Input: dimensioned drawing with shaded views. Units: mm. Origin: part minimum x, y, z. Coordinates: 2 decimals unless noted, no trailing zeros. Order: outer loops, then holes, each group sorted by start corner. A loop starts at its lowest first (then second) coordinate and runs counter-clockwise, first axis right, second up. Notation, with made-up numbers: (87, -10.75) - (104, -10.75) arc R24 ccw to (104, 26.25) - close; hole circle Ø5 at (-33.5, 8). An arc over 180 degrees is marked (long way). One line per question, with ' | ' between items. Start each with the question number.
(1) Section A-A (z = 19.5). Return the cut outline in (x, y).
(2) Section B-B (x = 19.5). Return the cut outline in (y, z), then the cut area to 3 significant figures.
(3) Draft query along Z for the marked faces 1, 2, 3 and 4. Return one class per face: +Z half, -Z half, draft (parallel to the pull), parting line (faces both ways), or undercut.
(4) Line query: line 1 along X through (y, z) = (21.5, 19.5); line 2 along X through (y, z) = (12, 6.5); line 3 along Z through (x, y) = (12.5, 22). Output: solid intervals per line, ascending.
(5) Section D-D (y = 3). Return the cut outline in (x, z).
(6) Section C-C (y = 11). Return the cut outline in (x, z).
(7) Contact query for flat-ended pins moving along their axis: P1, Ø1.5, axis at x = 32.5, z = 16, coming from the -Y side; P2, Ø6, axis at y = 6, z = 14.5, coming from the -X side; P3, Ø4, axis at x = 19, z = 21, coming from the +Y side. Output: stop coordinate, or through.
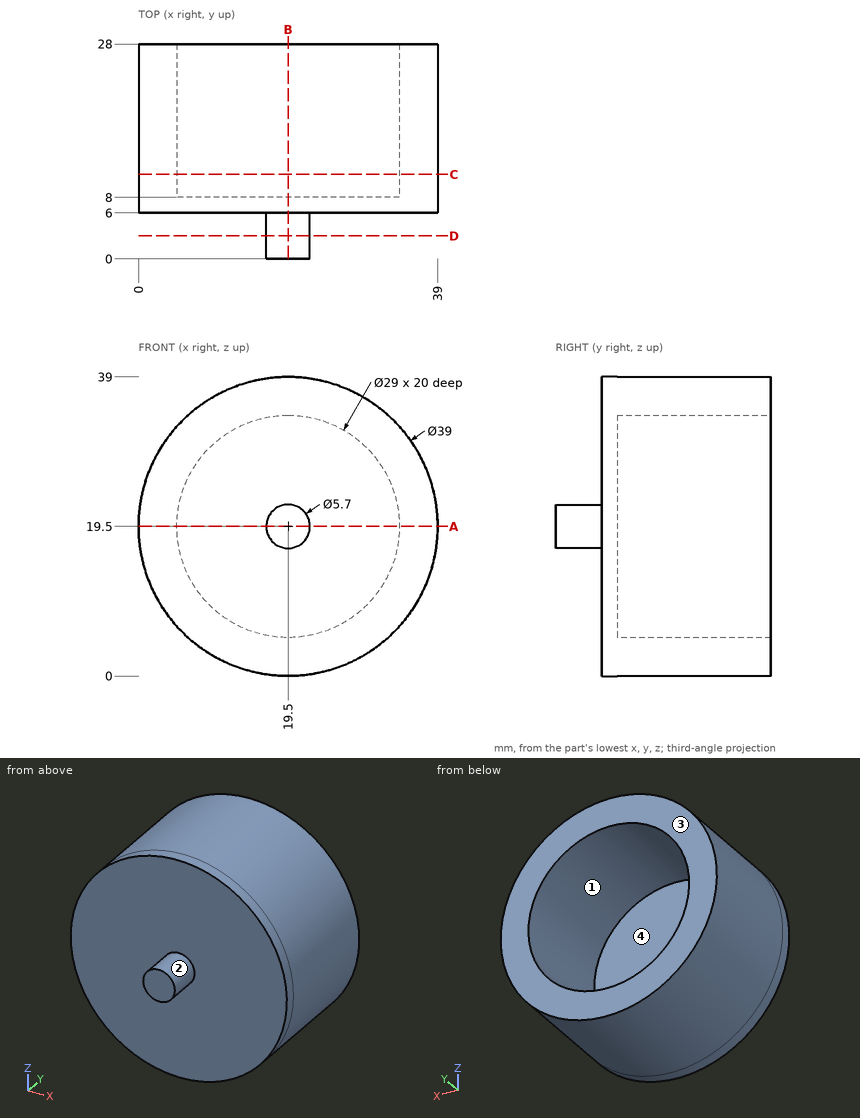
Response values:
1) outline: (0, 6) - (16.65, 6) - (16.65, 0) - (22.35, 0) - (22.35, 6) - (39, 6) - (39, 28) - (34, 28) - (34, 8) - (5, 8) - (5, 28) - (0, 28) - close
2) outline: (0, 16.65) - (6, 16.65) - (6, 0) - (28, 0) - (28, 5) - (8, 5) - (8, 34) - (28, 34) - (28, 39) - (6, 39) - (6, 22.35) - (0, 22.35) - close | area: 312 mm²
3) face 1: undercut | face 2: parting line | face 3: draft | face 4: undercut
4) line 1: x = 0 to 5, 34 to 39 | line 2: x = 4.97 to 13.08, 25.92 to 34.03 | line 3: z = 1.3 to 6.8, 32.2 to 37.7
5) outline: circle Ø5.7 at (19.5, 19.5)
6) outline: circle Ø39 at (19.5, 19.5); hole circle Ø29 at (19.5, 19.5)
7) P1: stops at y = 6 | P2: stops at x = 0.1 | P3: stops at y = 8
